Source: CAD feature listing. Evaluate the final solid. Frame: model axes, mm. A direction names the side the tool comes from. Coordinates: 2 decimals unless noted, no trailing zeros. Loops run counter-clockwise (first coordinate to the right, second up) from the corner with the lowest first, then second, coordinate; pieces in that order, holes last.
```python
from build123d import *

# Parameters (mm, degrees)
BOSS_EXTRUDE1_DEPTH = 11
SKETCH2_R           = 1.45
CUT_EXTRUDE1_DEPTH  = 8
SKETCH3_R           = 1.5
CUT_EXTRUDE2_DEPTH  = 10
CUT_EXTRUDE4_START  = -2
CUT_EXTRUDE4_DEPTH  = 2.4
SKETCH1_4_W         = 4.95
SKETCH1_4_H         = 8.65
SKETCH1_4_W_2       = 3.45
BOSS_EXTRUDE2_DEPTH = 11
CUT_EXTRUDE3_START  = -2
SKETCH5_R           = 1.5
CUT_EXTRUDE3_DEPTH  = 2.4
FILLET2_R           = 0.5


with BuildPart() as part:
    # Sketch1 → Boss-Extrude1 (new body)
    with BuildSketch(Plane(origin=(0, 0, 0), x_dir=(1, 0, 0), z_dir=(0, 1, 0))):
        with BuildLine():
            ThreePointArc((-1.55, 10), (0, 8.45), (1.55, 10))
            Line((1.55, 10), (10.4, 10))
            Line((10.4, 10), (10.4, -10))
            Line((10.4, -10), (-10.4, -10))
            Line((-10.4, -10), (-10.4, 10))
            Line((-10.4, 10), (-1.55, 10))
        make_face()
    extrude(amount=BOSS_EXTRUDE1_DEPTH)

    # Sketch2 → Cut-Extrude1 (cut)
    with BuildSketch(Plane.XY.offset(10)):
        with Locations((-5.9, 5.5)):
            Circle(SKETCH2_R)
        with Locations((6.1, 5.5)):
            Circle(SKETCH2_R)
    extrude(amount=-CUT_EXTRUDE1_DEPTH, mode=Mode.SUBTRACT)

    # Sketch3 → Cut-Extrude2 (cut)
    with BuildSketch(Plane(origin=(0, 0, -10), x_dir=(-1, 0, 0), z_dir=(0, 0, -1))):
        with Locations((-8.1, 5.5)):
            Circle(SKETCH3_R)
        with Locations((8.1, 5.5)):
            Circle(SKETCH3_R)
    extrude(amount=-CUT_EXTRUDE2_DEPTH, mode=Mode.SUBTRACT)

    # Sketch6 → Cut-Extrude4 (cut)
    with BuildSketch(Plane.XY.offset(10).offset(CUT_EXTRUDE4_START)):
        Polygon((-5.9, 8.559956427), (-8.55, 7.029978213), (-8.55, 3.970021787), (-8.55, 0), (-3.25, 0), (-3.25, 3.970021787), (-3.25, 7.029978213), align=None)
        Polygon((6.1, 8.559956427), (3.45, 7.029978213), (3.45, 3.970021787), (3.45, 0), (8.75, 0), (8.75, 3.970021787), (8.75, 7.029978213), align=None)
    extrude(amount=-CUT_EXTRUDE4_DEPTH, mode=Mode.SUBTRACT)

    # Sketch1<4> → Boss-Extrude2 (add, through all)
    with BuildSketch(Plane(origin=(0, 0, 0), x_dir=(1, 0, 0), z_dir=(0, 1, 0))):
        with Locations((12.875, 5.675)):
            Rectangle(SKETCH1_4_W, SKETCH1_4_H)
        with Locations((-12.125, 5.675)):
            Rectangle(SKETCH1_4_W_2, SKETCH1_4_H)
    extrude(amount=BOSS_EXTRUDE2_DEPTH)

    # Sketch5 → Cut-Extrude3 (cut)
    # profile 1 of 2: a face of its own
    with BuildSketch(Plane(origin=(0, 0, -10), x_dir=(-1, 0, 0), z_dir=(0, 0, -1)).offset(CUT_EXTRUDE3_START)):
        Polygon((-5.475, 0), (-5.475, 3.984455543), (-5.475, 7.015544457), (-8.1, 8.531088913), (-10.725, 7.015544457), (-10.725, 3.984455543), (-10.725, 0), align=None)
        with Locations((-8.1, 5.5)):
            Circle(SKETCH5_R, mode=Mode.SUBTRACT)
    # profile 2 of 2: a face of its own
    with BuildSketch(Plane(origin=(0, 0, -10), x_dir=(-1, 0, 0), z_dir=(0, 0, -1)).offset(CUT_EXTRUDE3_START)):
        Polygon((5.475, 0), (10.725, 0), (10.725, 3.984455543), (10.725, 7.015544457), (8.1, 8.531088913), (5.475, 7.015544457), (5.475, 3.984455543), align=None)
    extrude(amount=-CUT_EXTRUDE3_DEPTH, mode=Mode.SUBTRACT)

    # Fillet2
    fillet2_edges = [part.edges().sort_by_distance(p)[0] for p in [
        (1.55, 5.5, -10),
        (10.4, 5.5, 10),
        (-10.4, 5.5, 10),
        (-1.55, 5.5, -10),
        (10.4, 5.5, -1.35),
        (15.35, 5.5, -1.35),
        (15.35, 5.5, -10),
        (-13.85, 5.5, -10),
        (-13.85, 5.5, -1.35),
        (-10.4, 5.5, -1.35),
    ]]
    fillet(fillet2_edges, radius=FILLET2_R)


solid = part.part
```
Q1. First-contact query: pin 1 Ø0.7 at (y, z) = (4.5, 6.5) entering from -X; pin 2 Ø5 at (x, y) = (11, 6.5) entering from +Z; pin 3 Ø2.5 at (x, y) = (-12, 7) entering from +Z; pin 4 Ø1.5 at (y, z) = (9, -1) entering from -X. Flat tips, straight axial feed; report the tip coordinate or a pass-through.
Q2. Reachability of faces 4 (the flat face through (-6, 6, 2)), 5 (the flat face through (8, 6, 0)), 6 (the flat face through (-5.475, 4, -7)) from +Z, -Z, +X, -X, +Y, -Y: full face, straight path, thin tool, end or side. Return the list, or none.
Q3. Section query D-D on y = 1.25. Count the separate pieces of the cut face and the enclosed holes in it, then the cut area to 3 significant figures.
Q4. Section query C-C on z = -7.25. Return the cut outline in (x, y) (3 decimals).
Q5. Section query B-B on y = 9. Return the cut outline in (x, z).
Q6. Section query A-A on z = 3.75. Return the cut outline in (x, y).
Q7. Material intervals for line 1 along Z through (x, y) = (-7.5, 7.5); line 2 along Z through (x, y) = (4.5, 4); line 3 along X through (y, z) = (6.5, 7.5), sorted ascending.
Q8. Draft query along Y for faces 1 (the cylindrical face through (-9.486, 4.925, -9.014)), 2 (the flat face through (-7.206, 7.806, 6.817)), 3 (the flat face through (-6, 3, 5.6)). Return one class per face: released by +Y, released by -Y, zero draft, split by the parting line, or undercut.
Resolved:
1. pin 1: stops at x = -10.4
1. pin 2: stops at z = 10
1. pin 3: stops at z = -1.33
1. pin 4: stops at x = -13.84
2. face 4: +Z
2. face 5: -Z
2. face 6: -Y
3. separate pieces: 1
3. enclosed holes: 4
3. area: 434 mm2
4. outline: (-13.85, 0) - (-10.725, 0) - (-10.725, 7.016) - (-8.1, 8.531) - (-5.475, 7.016) - (-5.475, 0) - (5.475, 0) - (5.475, 7.016) - (8.1, 8.531) - (10.725, 7.016) - (10.725, 0) - (15.35, 0) - (15.35, 11) - (-13.85, 11) - close
5. outline: (-13.85, -9.5) arc R0.5 ccw to (-13.35, -10) - (-1.99, -10) arc R0.5 ccw to (-1.5, -9.62) arc R1.55 cw to (1.5, -9.62) arc R0.5 ccw to (1.99, -10) - (14.85, -10) arc R0.5 ccw to (15.35, -9.5) - (15.35, -1.85) arc R0.5 ccw to (14.85, -1.35) - (10.9, -1.35) arc R0.5 cw to (10.4, -0.85) - (10.4, 9.5) arc R0.5 ccw to (9.9, 10) - (-9.9, 10) arc R0.5 ccw to (-10.4, 9.5) - (-10.4, -0.85) arc R0.5 cw to (-10.9, -1.35) - (-13.35, -1.35) arc R0.5 ccw to (-13.85, -1.85) - close
6. outline: (-10.4, 0) - (10.4, 0) - (10.4, 11) - (-10.4, 11) - close; hole circle Ø2.9 at (-5.9, 5.5); hole circle Ø2.9 at (6.1, 5.5)
7. line 1: z = -10 to -8, -5.6 to 5.6, 8 to 10
7. line 2: z = -10 to 5.6, 8 to 10
7. line 3: x = -10.4 to -8.55, -3.25 to 3.45, 8.75 to 10.4
8. face 1: undercut
8. face 2: released by -Y
8. face 3: zero draft
